Could you check a few things on this model? Use its own coordinates, in mm. Round coordinates to 2 decimals unless told otherwise and drop trailing zeros. Loops run counter-clockwise (first coordinate to the right, second up) from the corner with the lowest first, then second, coordinate; pieces in that order, holes last. Notation, with made-up numbers: M 56,-33 L 67,-33 A18 ccw 67,-27 Z; hole C 34,-30.5 d10. An arc over 180 degrees is marked long. One line per item, written item: value. Start each with the question number.
Q1. Please list where these lines run through material, in increasing order: line 1 along X through (y, z) = (271.5, 5.25); line 2 along Y through (x, z) = (221, 1); line 3 along Y through (x, z) = (371, 10).
Q2. Imagine slicing it at C-C (z = 2). Please give me the cut outline in (x, y).
Q3. Imagine slicing it at A-A (y = 160). Please give me the cut outline in (x, z).
Q4. Imagine slicing it at B-B (x = 250). Please give me the cut outline in (y, z).
Q5. Imagine slicing it at D-D (y = 572). Please give me the cut outline in (x, z).
Q6. I'm going to push flat-ended pins straight in: pin 1 Ø6 at (x, z) = (211.5, 7.5) entering from +Y; pin 2 Ø6 at (y, z) = (610, 9.5) entering from +X; pin 3 Ø0.6 at (x, z) = (499.5, 4) entering from +Y. Where does each tip first touch, or does it pass through?
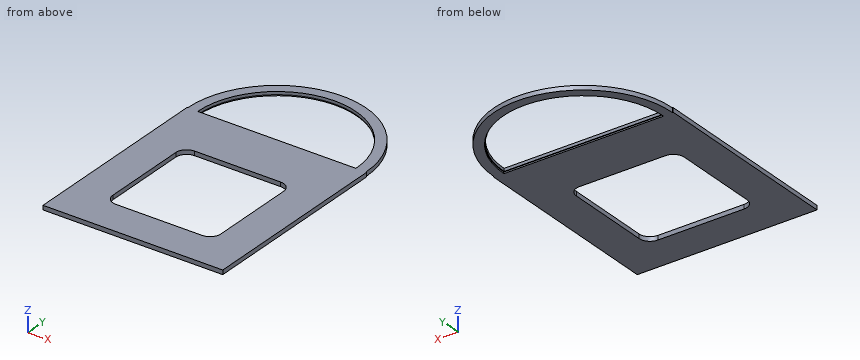
Solid Edge part; units mm, degrees
sketch "Sketch1" plane through (0, 0, 0) normal (0, 0, 1) x (1, 0, 0)
  line L0 (0, 0) -> (500, 0)
  line L1 (500, 0) -> (500, 550)
  arc A0 (0, 550) -> (500, 550) centre (250, 550) cw
  line L2 (0, 550) -> (0, 0)
extrude "Protrusion1" add sketch "Sketch1" along normal blind 12
sketch "Sketch2" plane through (250, 400, 12) normal (0, 0, 1) x (1, 0, 0)
  line L0 (-120, -300) -> (120, -300)
  arc A0 (150, -270) -> (120, -300) centre (120, -270) cw
  line L1 (150, -270) -> (150, -30)
  arc A1 (120, 0) -> (150, -30) centre (120, -30) cw
  line L2 (120, 0) -> (-120, 0)
  arc A2 (-150, -30) -> (-120, 0) centre (-120, -30) cw
  line L3 (-150, -30) -> (-150, -270)
  arc A3 (-120, -300) -> (-150, -270) centre (-120, -270) cw
  dimension "D1" = 150
extrude "Boxenloch" cut sketch "Sketch2" against normal blind 429.6561
sketch "Sketch3" plane through (250, 400, 0) normal (0, 0, -1) x (-1, 0, 0)
  line L0 (-220, 150) -> (220, 150)
  arc A0 (-220, 150) -> (220, 150) centre (0, 150) cw
extrude "Ausschnitt_4" cut sketch "Sketch3" against normal blind 186.1515
sketch "Sketch4" plane through (250, 400, 0) normal (0, 0, -1) x (-1, 0, 0)
  arc A0 (222, 150) -> (-222, 150) centre (0, 150) ccw
  line L0 (-222, 150) -> (-222, 148)
  line L1 (-222, 148) -> (222, 148)
  line L2 (222, 150) -> (222, 148)
  dimension "D1" = 222
extrude "Ausschnitt_5" cut sketch "Sketch4" against normal blind 4
sketch "Sketch5" plane through (250, 400, 0) normal (0, 0, -1) x (-1, 0, 0)
  line L0 (250, 150) -> (248, 150)
  arc A0 (-248, 150) -> (248, 150) centre (0, 150) cw
  line L1 (-250, 150) -> (-248, 150)
  arc A1 (250, 150) -> (-250, 150) centre (0, 150) ccw
extrude "Ausschnitt_6" cut sketch "Sketch5" against normal blind 184.2167
Report:
1. line 1: x = 0 to 100, 400 to 500
1. line 2: y = 0 to 100, 400 to 548, 770.1 to 796.3
1. line 3: y = 0 to 100.02, 399.98 to 550, 733.74 to 766.48
2. outline: M 0,0 L 500,0 L 500,550 L 498,550 A248 ccw 2,550 L 0,550 Z; hole M 28,548 L 472,548 L 472,550 A222 ccw 28,550 Z; hole M 100,130 A30 ccw 130,100 L 370,100 A30 ccw 400,130 L 400,370 A30 ccw 370,400 L 130,400 A30 ccw 100,370 Z
3. outline: M 0,0 L 100,0 L 100,12 L 0,12 Z; M 400,0 L 500,0 L 500,12 L 400,12 Z
4. outline: M 0,0 L 100,0 L 100,12 L 0,12 Z; M 400,0 L 548,0 L 548,4 L 550,4 L 550,12 L 400,12 Z; M 770,4 L 772,4 L 772,0 L 798,0 L 798,12 L 770,12 Z
5. outline: M 2.98,0 L 29.09,0 L 29.09,4 L 31.1,4 L 31.1,12 L 2.98,12 Z; M 468.9,4 L 470.91,4 L 470.91,0 L 497.02,0 L 497.02,12 L 468.9,12 Z
6. pin 1: stops at y = 795.45
6. pin 2: stops at x = 491.36
6. pin 3: stops at y = 550
